Part print with two shaded views. Sizes in mm from the minimum x, y, z corner. Give positions to 0.01 mm unless a question says otherwise; leave off trailing zeros. Write each loop counter-clockwise with the first axis right and the second up, starting at its lowest first coordinate (ties: lowest second). Pieces come first, ordered by that corner, then holes. Notation, with made-up numbers: (-6, 37) - (12, 37) arc R10 cw to (12, 42) - close; hole circle Ø7 at (80.25, 84). An arc over 180 degrees is marked (long way). One line per item, written item: value. Start each with the question number.
(1) Mould opens along X. For the marked faces 1 and 2 say: pulls with the +X half, pulls with the -X half, needs draft (parallel to the pull), parting line crosses it, or undercut.
(2) Drop flat-ended pins along their axis: P1, Ø1.2, axis at x = 3, z = 5, coming from the +Y side; P2, Ø1.2, axis at x = 1, z = 5, coming from the -Y side; P3, Ø5, axis at x = 145.5, y = 42, coming from the +Z side. Give the stop position or say it passes through.
(3) Probe L1, parallel to X at y = 80.5, z = 6; L2, parallel to Z at x = 145.5, y = 39. List the from-to ranges inside material, lowest first.
(4) Cut at B-B, the plane y = 55.5. List the corners of the cut face in (x, z), and give its area (3 significant figures).
(5) Cut at A-A, the plane z = 6.5. List the corners of the cut face in (x, y).
(6) Cut at C-C, the plane x = 54. List the corners of the cut face in (y, z).
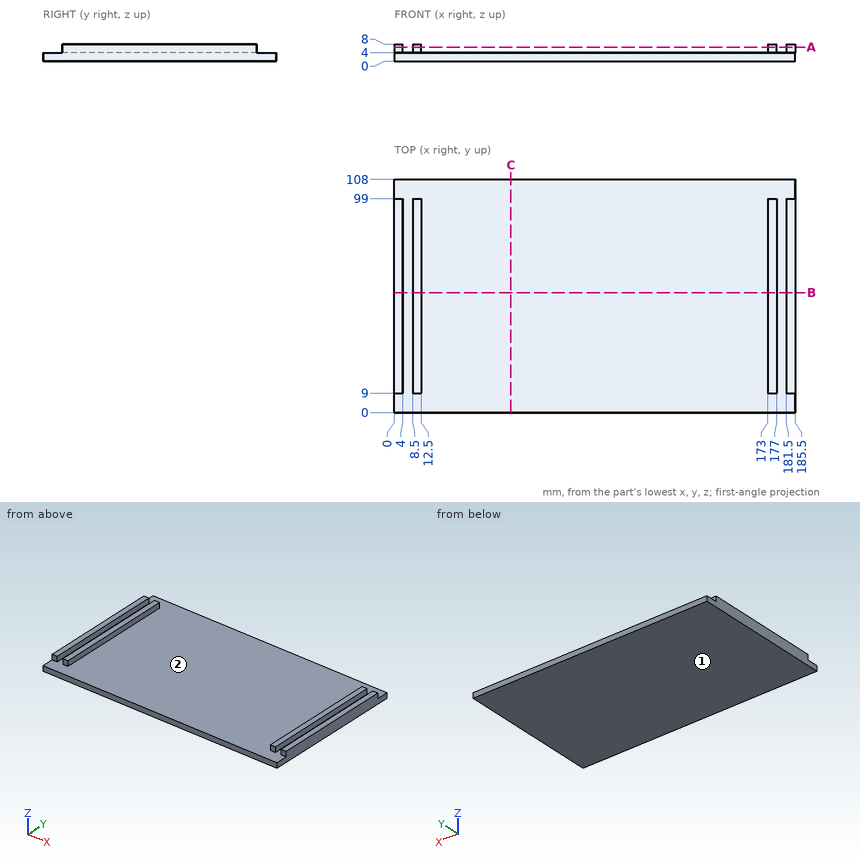
Answers follow:
1. face 1: needs draft
1. face 2: undercut
2. P1: stops at y = 99
2. P2: stops at y = 9
2. P3: stops at z = 4
3. L1: x = 0 to 4, 8.5 to 12.5, 173 to 177, 181.5 to 185.5
3. L2: z = 0 to 4
4. outline: (0, 0) - (185.5, 0) - (185.5, 8) - (181.5, 8) - (181.5, 4) - (177, 4) - (177, 8) - (173, 8) - (173, 4) - (12.5, 4) - (12.5, 8) - (8.5, 8) - (8.5, 4) - (4, 4) - (4, 8) - (0, 8) - close
4. area: 806 mm²
5. outline: (0, 9) - (4, 9) - (4, 99) - (0, 99) - close; (8.5, 9) - (12.5, 9) - (12.5, 99) - (8.5, 99) - close; (173, 9) - (177, 9) - (177, 99) - (173, 99) - close; (181.5, 9) - (185.5, 9) - (185.5, 99) - (181.5, 99) - close
6. outline: (0, 0) - (108, 0) - (108, 4) - (0, 4) - close
